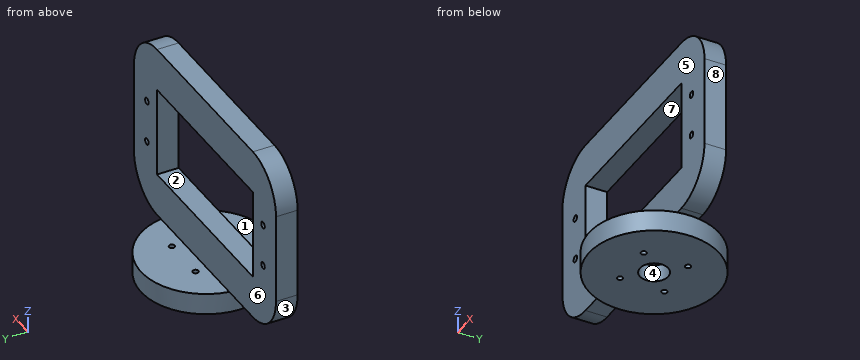
from build123d import *

# Parameters (mm, degrees)
SKETCH1_W           = 61.5
SKETCH1_H           = 30
BOSS_EXTRUDE2_DEPTH = 5
SKETCH2_W           = 61.5
SKETCH2_H           = 5
BOSS_EXTRUDE3_DEPTH = 41
SKETCH3_W           = 41.5
SKETCH3_H           = 21
CUT_EXTRUDE1_DEPTH  = 5
SKETCH4_OUTSIDE_W   = 79.99
SKETCH4_OUTSIDE_H   = 48.49
SKETCH4_OUTSIDE_R   = 15
CUT_EXTRUDE2_DEPTH  = 5
SKETCH5_R           = 3.25
CUT_EXTRUDE5_DEPTH  = 4
FILLET1_R           = 10
FILLET2_R           = 10
FILLET3_R           = 10
FILLET4_R           = 10
SKETCH7_R           = 0.75
CUT_EXTRUDE7_DEPTH  = 5
SKETCH8_R           = 0.65
CUT_EXTRUDE8_DEPTH  = 5


with BuildPart() as part:
    # Sketch1 → Boss-Extrude2 (new body)
    with BuildSketch(Plane.XY):
        with Locations((-30.75, 15)):
            Rectangle(SKETCH1_W, SKETCH1_H)
    extrude(amount=BOSS_EXTRUDE2_DEPTH)

    # Sketch2 → Boss-Extrude3 (add)
    with BuildSketch(Plane.XY.offset(5)):
        with Locations((-30.75, 15)):
            Rectangle(SKETCH2_W, SKETCH2_H)
    extrude(amount=BOSS_EXTRUDE3_DEPTH)

    # Sketch3 → Cut-Extrude1 (cut)
    with BuildSketch(Plane.XZ.offset(-12.5)):
        with Locations((-30.75, 25.5)):
            Rectangle(SKETCH3_W, SKETCH3_H)
    extrude(amount=-CUT_EXTRUDE1_DEPTH, mode=Mode.SUBTRACT)

    # Sketch4 outside → Cut-Extrude2 (cut)
    with BuildSketch(Plane(origin=(0, 0, 0), x_dir=(-1, 0, 0), z_dir=(0, 0, -1))):
        with Locations((30.75, 15)):
            Rectangle(SKETCH4_OUTSIDE_W, SKETCH4_OUTSIDE_H)
        with Locations((26.5, 15)):
            Circle(SKETCH4_OUTSIDE_R, mode=Mode.SUBTRACT)
    extrude(amount=-CUT_EXTRUDE2_DEPTH, mode=Mode.SUBTRACT)

    # Sketch5 → Cut-Extrude5 (cut)
    with BuildSketch(Plane(origin=(0, 0, 0), x_dir=(-1, 0, 0), z_dir=(0, 0, -1))):
        with Locations((26.5, 15)):
            Circle(SKETCH5_R)
    extrude(amount=-CUT_EXTRUDE5_DEPTH, mode=Mode.SUBTRACT)

    # Fillet1
    fillet1_edges = [part.edges().sort_by_distance(p)[0] for p in [
        (-61.5, 15, 5),
    ]]
    fillet(fillet1_edges, radius=FILLET1_R)

    # Fillet2
    fillet2_edges = [part.edges().sort_by_distance(p)[0] for p in [
        (-61.5, 15, 46),
    ]]
    fillet(fillet2_edges, radius=FILLET2_R)

    # Fillet3
    fillet3_edges = [part.edges().sort_by_distance(p)[0] for p in [
        (0, 15, 5),
    ]]
    fillet(fillet3_edges, radius=FILLET3_R)

    # Fillet4
    fillet4_edges = [part.edges().sort_by_distance(p)[0] for p in [
        (0, 15, 46),
    ]]
    fillet(fillet4_edges, radius=FILLET4_R)

    # Sketch7 → Cut-Extrude7 (cut)
    with BuildSketch(Plane.XZ.offset(-12.5)):
        with Locations((-55.9, 20.5)):
            Circle(SKETCH7_R)
        with Locations((-55.9, 30.5)):
            Circle(SKETCH7_R)
        with Locations((-5.6, 30.5)):
            Circle(SKETCH7_R)
        with Locations((-5.6, 20.5)):
            Circle(SKETCH7_R)
    extrude(amount=-CUT_EXTRUDE7_DEPTH, mode=Mode.SUBTRACT)

    # Sketch8 → Cut-Extrude8 (cut)
    with BuildSketch(Plane(origin=(0, 0, 0), x_dir=(-1, 0, 0), z_dir=(0, 0, -1))):
        with Locations((31.626524164, 20.126524164)):
            Circle(SKETCH8_R)
        with Locations((31.626524164, 9.873475836)):
            Circle(SKETCH8_R)
        with Locations((21.373475836, 9.873475836)):
            Circle(SKETCH8_R)
        with Locations((21.373475836, 20.126524164)):
            Circle(SKETCH8_R)
    extrude(amount=-CUT_EXTRUDE8_DEPTH, mode=Mode.SUBTRACT)


solid = part.part
Verification items for the finished model (mm, model axes). Face numbers are marked on the shaded views. A direction names the side the tool comes from. Coordinates: 2 decimals unless noted, no trailing zeros. Order: outer loops, then holes, each group sorted by start corner. A loop starts at its lowest first (then second) coordinate and runs counter-clockwise, first axis right, second up. Notation, with made-up numbers: (82.5, 26) -> (131.5, 26) arc R19 ccw to (131.5, 32) -> close; hole circle Ø8 at (12.5, 44). An arc over 180 degrees is marked (long way). Put each result on its own line as item: value. Start each with the question number.
1. Material ranges on L1, parallel to Z at x = -55.9, y = 15.05; L2, parallel to X at y = 16, z = 17.5; L3, parallel to Y at x = -5, z = 11, recorded low to high. Write a range as [from, to].
2. Mould release check, pull along Z, two halves, no side actions. Record for the marked faces 1, 2, 3 and 4: released by +Z, released by -Z, zero draft, split by the parting line, or undercut.
3. Access from +Z, -Z, +X, -X, +Y, -Y to the whole of each face (thin tool, end or side, straight path). Record for the marked faces 5, 6, 7 and 8.
4. Cross-section at A-A, the plane y = 15. Record the boundary of the cut face in (x, z).
5. Cross-section at C-C, the plane x = -20. Record the boundary of the cut face in (y, z).
6. Go/stop test with flat-tipped pins: pin 1 Ø12 at (y, z) = (22.5, 5.5) entering from -X; pin 2 Ø8 at (x, z) = (-47.5, 11.5) entering from -Y; pin 3 Ø1.5 at (x, y) = (-21.37, 20.13) entering from +Z. Record where each tip stops, or that it passes through.
7. Cross-section at B-B, the plane z = 16.5. Record the boundary of the cut face in (x, y).
8. Cross-section at D-D, the plane x = -8. Record the boundary of the cut face in (y, z), then the cut area to 3 significant figures.
Computed:
1. L1: [6.02, 19.75], [21.25, 29.75], [31.25, 44.98]
1. L2: [-61.5, -51.5], [-10, 0]
1. L3: [12.5, 17.5]
2. face 1: released by +Z
2. face 2: undercut
2. face 3: released by -Z
2. face 4: zero draft
3. face 5: +Z, +X, -X, -Y
3. face 6: +Z, +X, -X, +Y
3. face 7: +Y, -Y
3. face 8: +Z, -Z, +X, +Y, -Y
4. outline: (-61.5, 15) arc R10 ccw to (-51.5, 5) -> (-41.5, 5) -> (-41.5, 0) -> (-29.75, 0) -> (-29.75, 4) -> (-23.25, 4) -> (-23.25, 0) -> (-11.5, 0) -> (-11.5, 5) -> (-10, 5) arc R10 ccw to (0, 15) -> (0, 36) arc R10 ccw to (-10, 46) -> (-51.5, 46) arc R10 ccw to (-61.5, 36) -> close; hole circle Ø1.5 at (-55.9, 20.5); hole circle Ø1.5 at (-55.9, 30.5); hole (-51.5, 15) -> (-10, 15) -> (-10, 36) -> (-51.5, 36) -> close; hole circle Ø1.5 at (-5.6, 20.5); hole circle Ø1.5 at (-5.6, 30.5)
5. outline: (1.48, 0) -> (28.52, 0) -> (28.52, 5) -> (17.5, 5) -> (17.5, 15) -> (12.5, 15) -> (12.5, 5) -> (1.48, 5) -> close; (12.5, 36) -> (17.5, 36) -> (17.5, 46) -> (12.5, 46) -> close
6. pin 1: x = -59.36
6. pin 2: y = 12.5
6. pin 3: z = 5
7. outline: (-61.5, 12.5) -> (-51.5, 12.5) -> (-51.5, 17.5) -> (-61.5, 17.5) -> close; (-10, 12.5) -> (0, 12.5) -> (0, 17.5) -> (-10, 17.5) -> close
8. outline: (12.5, 5.2) -> (17.5, 5.2) -> (17.5, 45.8) -> (12.5, 45.8) -> close
8. area: 203 mm2
